Design review of the part built by this model. Coordinates are the model's own, in mm. A direction names the side the tool comes from. Give positions to 0.01 mm unless a question says otherwise; leave off trailing zeros. Order: outer loops, then holes, each group sorted by start corner. A loop starts at its lowest first (then second) coordinate and runs counter-clockwise, first axis right, second up. Notation, with made-up numbers: M -5.5,39.25 L 22.5,39.25 A20 cw 22.5,44.25 Z; hole C 79,53 d4. An arc over 180 degrees is marked long. Answer as a JSON object with one key per item and string values.
from build123d import *

# Parameters (mm, degrees)
SKETCH_1_W          = 10
SKETCH_1_H          = 10
SKETCH_1_W_2        = 8
SKETCH_1_H_2        = 8
EXTRUDE_1_DEPTH     = 95
SKETCH_2_R          = 1.6
CUT_EXTRUDE_1_DEPTH = 96.655632349
SKETCH_3_R          = 1.6
CUT_EXTRUDE_2_DEPTH = 96.655632349


with BuildPart() as part:
    # ｽｹｯﾁ1 → ﾎﾞｽ - 押し出し1 (new body)
    with BuildSketch(Plane.XY):
        Rectangle(SKETCH_1_W, SKETCH_1_H)
        Rectangle(SKETCH_1_W_2, SKETCH_1_H_2, mode=Mode.SUBTRACT)
    extrude(amount=EXTRUDE_1_DEPTH)

    # ｽｹｯﾁ2 → ｶｯﾄ - 押し出し1 (cut, through all)
    with BuildSketch(Plane(origin=(0, 5, 0), x_dir=(1, 0, 0), z_dir=(0, 1, 0))):
        with Locations(Location((0, -5, 0), (0, 0, 270))):
            Circle(SKETCH_2_R)
        with Locations(Location((0, -80, 0), (0, 0, 270))):
            Circle(SKETCH_2_R)
        with Locations(Location((0, -19.5, 0), (0, 0, 270))):
            Circle(SKETCH_2_R)
    extrude(amount=-CUT_EXTRUDE_1_DEPTH, mode=Mode.SUBTRACT)

    # ｽｹｯﾁ3 → ｶｯﾄ - 押し出し2 (cut, through all)
    with BuildSketch(Plane.ZY.offset(5)):
        with Locations((15, 0)):
            Circle(SKETCH_3_R)
        with Locations((90, 0)):
            Circle(SKETCH_3_R)
    extrude(amount=-CUT_EXTRUDE_2_DEPTH, mode=Mode.SUBTRACT)


solid = part.part
(1) Tool access review of faces 1 (the cylindrical face through (4.49, 0.07, 88.4)), 2 (the flat face through (4, 0, 47)): name each direction out of +Z, -Z, +X, -X, +Y, -Y from which nothing blocks a thin tool from reaching the whole face with its end or side.
Checked values:
{"face 1": "+X, -X", "face 2": "+Z, -Z"}
(2) Draft analysis for pull direction Z (two halves, no side actions). For faces 3 (the flat face through (-4.5, 0.1, 0)), 4 (the flat face through (-4.5, 0.1, 95)), 5 (the flat face through (0, 4, 47)), 6 (the cylindrical face through (-0.61, -4.49, 6.48)), state which applies: +Z half, -Z half, draft (parallel to the pull), parting line (faces both ways), or undercut.
Checked values:
{"face 3": "-Z half", "face 4": "+Z half", "face 5": "draft", "face 6": "undercut"}
(3) We need section C-C (z = 65.5). Write out the cut boundary in (x, y).
Checked values:
{"outline": "M -5,-5 L 5,-5 L 5,5 L -5,5 Z; hole M -4,-4 L 4,-4 L 4,4 L -4,4 Z"}
(4) Insertion check: pin 1 (3 mm diameter, centred on x = 2, y = 2, fed in from -Z). The pin has a flat end and moves straight along its axis. Give the tip position at first contact, or say it passes through.
Checked values:
{"pin 1": "passes through"}
(5) We need section B-B (x = 0). Count the separate pieces of the cut face and the enclosed holes in it, plus the area to 3 significant figures.
Checked values:
{"separate pieces": "8", "enclosed holes": "0", "area": "171 mm^2"}
(6) We need section A-A (z = 5). Write out the cut boundary in (x, y).
Checked values:
{"outline": "M -5,-5 L -1.6,-5 L -1.6,-4 L -4,-4 L -4,4 L -1.6,4 L -1.6,5 L -5,5 Z; M 1.6,-5 L 5,-5 L 5,5 L 1.6,5 L 1.6,4 L 4,4 L 4,-4 L 1.6,-4 Z"}
(7) To check wall thickness, follow L1, parallel to X at y = 4.4, z = 80; L2, parallel to X at y = -2.5, z = 40. State the ranges of each line that lie inside material, in increasing order. Write a range as from..to.
Checked values:
{"L1": "x = -5..-1.6, 1.6..5", "L2": "x = -5..-4, 4..5"}
